from build123d import *

# Parameters (mm, degrees)
ESQUISSE1_W                    = 12.4
ESQUISSE1_H                    = 17.6
BOSS_EXTRU_1_DEPTH             = 7
ESQUISSE2_W                    = 0.5
ESQUISSE2_H                    = 0.5
BOSS_EXTRU_2_DEPTH             = 5.4
R_P_TITION_LIN_AIRE1_COUNT     = 3
R_P_TITION_LIN_AIRE1_PITCH     = 2.54
R_P_TITION_LIN_AIRE1_COL_COUNT = 3
R_P_TITION_LIN_AIRE1_COL_PITCH = 2.54


with BuildPart() as part:
    # Esquisse1 → Boss.-Extru.1 (new body)
    with BuildSketch(Plane.XY):
        with Locations((6.2, 8.8)):
            Rectangle(ESQUISSE1_W, ESQUISSE1_H)
    extrude(amount=BOSS_EXTRU_1_DEPTH)

    # Esquisse2 → Boss.-Extru.2 (add)
    with BuildSketch(Plane(origin=(0, 0, 0), x_dir=(-1, 0, 0), z_dir=(0, 0, -1))):
        with Locations((-6.2, 1.18)):
            Rectangle(ESQUISSE2_W, ESQUISSE2_H)
        with Locations((-6.2, 16.42)):
            Rectangle(ESQUISSE2_W, ESQUISSE2_H)
    boss_extru_2 = extrude(amount=BOSS_EXTRU_2_DEPTH)

    # Répétition linéaire1: Boss.-Extru.2 ×3
    with Locations(*[(i * R_P_TITION_LIN_AIRE1_PITCH, 0, 0) for i in range(1, R_P_TITION_LIN_AIRE1_COUNT)]):
        add(boss_extru_2)

    # Répétition linéaire1 col: Boss.-Extru.2 ×3
    with Locations(*[(-i * R_P_TITION_LIN_AIRE1_COL_PITCH, 0, 0) for i in range(1, R_P_TITION_LIN_AIRE1_COL_COUNT)]):
        add(boss_extru_2)


solid = part.part
Verification items for the finished model (mm, model axes). Round coordinates to 2 decimals unless told otherwise and drop trailing zeros. Write each loop counter-clockwise with the first axis right and the second up, starting at its lowest first coordinate (ties: lowest second). Pieces come first, ordered by that corner, then holes.
(1) Mould release check, pull along Y, two halves, no side actions. Record for faces 1 (the flat face through (6, 17.6, 3)), 2 (the flat face through (6, 9, 0)), 3 (the flat face through (6, 0, 3)): pulls with the +Y half, pulls with the -Y half, needs draft (parallel to the pull), parting line crosses it, or undercut.
Returned:
face 1: pulls with the +Y half
face 2: undercut
face 3: pulls with the -Y half
(2) Material ranges on line 1 (Y direction, x = 6, z = -1.25); line 2 (Z direction, x = 4.5, y = 9.5), recorded low to high.
Returned:
line 1: y = 0.93 to 1.43, 16.17 to 16.67
line 2: z = 0 to 7
(3) Section check C-C (y = 8). Enter the section's corners in (x, z), plus the area to 3 significant figures.
Returned:
outline: (0, 0) - (12.4, 0) - (12.4, 7) - (0, 7) - close
area: 86.8 mm2
(4) Section check A-A (z = -2). Give the number of separate pieces and of enclosed holes in the cut face, plus the area to 3 significant figures.
Returned:
separate pieces: 10
enclosed holes: 0
area: 2.50 mm2
(5) Section check B-B (x = 8.25). Enter the section's corners in (y, z).
Returned:
outline: (0, 0) - (17.6, 0) - (17.6, 7) - (0, 7) - close
(6) Depth check by flat-ended pin: pin 1 Ø0.6 at (y, z) = (16.5, -2.5) entering from +X; pin 2 Ø0.6 at (x, z) = (6, -2.5) entering from -Y; pin 3 Ø0.6 at (x, z) = (1, -2) entering from +Y. Enter the tip coordinate at first touch or a pass-through.
Returned:
pin 1: stops at x = 11.53
pin 2: stops at y = 0.93
pin 3: stops at y = 16.67
